```python
from build123d import *

# Parameters (mm, degrees)
SKETCH_1_W          = 36
SKETCH_1_H          = 36
EXTRUDE_1_DEPTH     = 10
SKETCH_2_W          = 20
SKETCH_2_H          = 20
EXTRUDE_2_DEPTH     = 3
SKETCH_3_R          = 5.5
EXTRUDE_4_DEPTH     = 10
SKETCH_4_R          = 1.5
CUT_EXTRUDE_1_DEPTH = 1
CUT_EXTRUDE_START   = -1
SKETCH_5_R          = 1.5
CUT_EXTRUDE_2_DEPTH = 1
FILLET_1_R          = 2
FILLET_2_R          = 1


with BuildPart() as part:
    # 草图1 → 凸台-拉伸1 (new body)
    with BuildSketch(Plane(origin=(0, 0, 0), x_dir=(1, 0, 0), z_dir=(0, 1, 0))):
        Rectangle(SKETCH_1_W, SKETCH_1_H)
    extrude(amount=-EXTRUDE_1_DEPTH)

    # 草图2 → 凸台-拉伸2 (add)
    with BuildSketch(Plane(origin=(0, 0, 0), x_dir=(1, 0, 0), z_dir=(0, 1, 0))):
        Rectangle(SKETCH_2_W, SKETCH_2_H)
    extrude(amount=EXTRUDE_2_DEPTH)

    # 草图3 → 凸台-拉伸4 (add)
    with BuildSketch(Plane(origin=(0, 3, 0), x_dir=(1, 0, 0), z_dir=(0, 1, 0))):
        with Locations(Location((0, 0, 0), (0, 0, 90))):
            Circle(SKETCH_3_R)
    extrude(amount=EXTRUDE_4_DEPTH)

    # 草图4 → 切除-拉伸1 (cut)
    with BuildSketch(Plane.ZY.offset(18)):
        with Locations((0, -5)):
            Circle(SKETCH_4_R)
    extrude(amount=-CUT_EXTRUDE_1_DEPTH, mode=Mode.SUBTRACT)

    # 草图5 → 切除-拉伸2 (cut)
    with BuildSketch(Plane(origin=(18, 0, 0), x_dir=(0, 0, -1), z_dir=(1, 0, 0)).offset(CUT_EXTRUDE_START)):
        with Locations(Location((0, -5, 0), (0, 0, 180))):
            Circle(SKETCH_5_R)
    extrude(amount=CUT_EXTRUDE_2_DEPTH, mode=Mode.SUBTRACT)

    # 圆角1
    fillet_1_edges = [part.edges().sort_by_distance(p)[0] for p in [
        (10, 3, 0),
        (0, 3, -10),
        (-10, 3, 0),
        (0, 3, 10),
        (0, 0, 18),
        (-18, 0, 0),
        (0, 0, -18),
        (18, 0, 0),
        (18, -5, 18),
        (-18, -5, 18),
        (-18, -5, -18),
        (18, -5, -18),
    ]]
    fillet(fillet_1_edges, radius=FILLET_1_R)

    # 圆角2
    fillet_2_edges = [part.edges().sort_by_distance(p)[0] for p in [
        (0, 13, 5.5),
    ]]
    fillet(fillet_2_edges, radius=FILLET_2_R)


solid = part.part
```
Here's how the part is built. I have some questions about the finished solid (model axes, mm). A direction names the side the tool comes from. Coordinates: 2 decimals unless noted, no trailing zeros. Order: outer loops, then holes, each group sorted by start corner. A loop starts at its lowest first (then second) coordinate and runs counter-clockwise, first axis right, second up. Notation, with made-up numbers: (70.25, 27) - (108.25, 27) arc R19 cw to (108.25, 59) - close; hole circle Ø7 at (45, 88). An arc over 180 degrees is marked (long way). One line per question, with ' | ' between items.
(1) Suppose I cut it at D-D on z = -7. List the corners of the cut face in (x, y) for me.
Report:
outline: (-18, -10) - (18, -10) - (18, -2) arc R2 ccw to (16, 0) - (10, 0) - (10, 1) arc R2 ccw to (8, 3) - (-8, 3) arc R2 ccw to (-10, 1) - (-10, 0) - (-16, 0) arc R2 ccw to (-18, -2) - close
(2) If we mould it in two halves opening along Z, with no side actions, what happens to faces 1 (the flat face through (10, 0.5, 0.1)), 2 (the flat face through (-17, -5, 0)), 3 (the cylindrical face through (-17.507, -3.513, -0.195)), 4 (the flat face through (-0.1, 0.5, 10))? For each: pulls with the +Z half, pulls with the -Z half, needs draft (parallel to the pull), parting line crosses it, or undercut.
Report:
face 1: needs draft | face 2: undercut | face 3: undercut | face 4: pulls with the +Z half
(3) Suppose I cut it at C-C on y = 10.25. List the corners of the cut face in (x, z) for me.
Report:
outline: circle Ø11 at (0, 0)
(4) If I drill on L1, parallel to Y at x = 8, z = -8; L2, parallel to Z at x = 17.2, y = -5; L3, parallel to Y at x = 17.8, z = 0, over which ranges is the centre line in solid material (lowest first)?
Report:
L1: y = -10 to 3 | L2: z = -17.6 to -1.5, 1.5 to 17.6 | L3: y = -10 to -6.5, -3.5 to -1.13
(5) For faces 5 (the flat face through (-0.1, 0.5, -10)), 6 (the cylindrical face through (17.49, -5.45, 1.43)), 7 (the flat face through (-1.9, 3, -5.4)), which set-ups out of +Z, -Z, +X, -X, +Y, -Y let a thin tool reach every point of the face, with its end or its side?
Report:
face 5: -Z, +X, -X, +Y | face 6: +X | face 7: +Y
(6) Suppose I cut it at B-B on z = 0. List the corners of the cut face in (x, y) for me, and give its area (3 significant figures).
Report:
outline: (-18, -10) - (18, -10) - (18, -6.5) - (17, -6.5) - (17, -3.5) - (18, -3.5) - (18, -2) arc R2 ccw to (16, 0) - (10, 0) - (10, 1) arc R2 ccw to (8, 3) - (5.5, 3) - (5.5, 12) arc R1 ccw to (4.5, 13) - (-4.5, 13) arc R1 ccw to (-5.5, 12) - (-5.5, 3) - (-8, 3) arc R2 ccw to (-10, 1) - (-10, 0) - (-16, 0) arc R2 ccw to (-18, -2) - (-18, -3.5) - (-17, -3.5) - (-17, -6.5) - (-18, -6.5) - close | area: 520 mm2
(7) Suppose I cut it at A-A on x = 6.5. List the corners of the cut face in (y, z) for me, and give its area (3 significant figures).
Report:
outline: (-10, -18) - (-2, -18) arc R2 ccw to (0, -16) - (0, -10) - (1, -10) arc R2 ccw to (3, -8) - (3, 8) arc R2 ccw to (1, 10) - (0, 10) - (0, 16) arc R2 ccw to (-2, 18) - (-10, 18) - close | area: 417 mm2
(8) Will these pins go through, and if not, where does the flat tip stop? pin 1 (0.8 mm diameter, centred on y = 0.5, z = 4, fed in from -X); pin 2 (0.5 mm diameter, centred on x = -2.5, y = 0.5, fed in from +Z); pin 3 (4 mm diameter, centred on x = 5, y = 7.5, fed in from +Z).
Report:
pin 1: stops at x = -10 | pin 2: stops at z = 10 | pin 3: stops at z = 4.61
